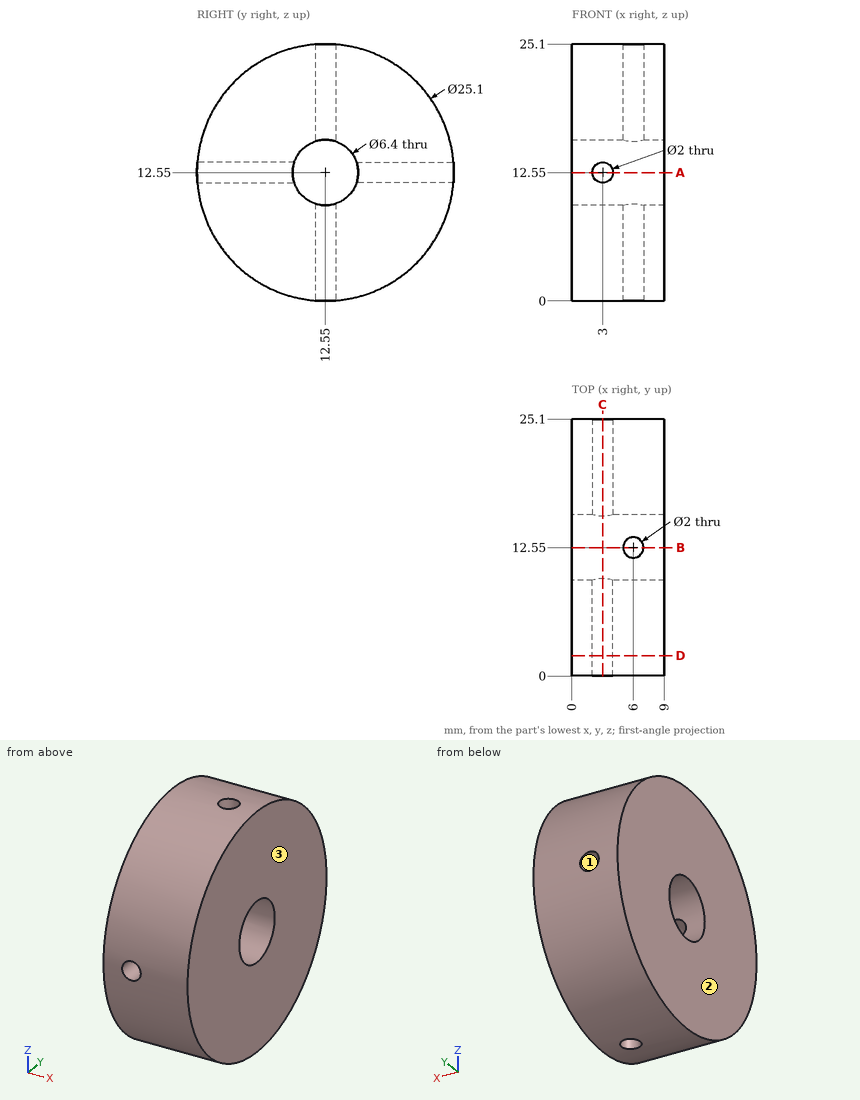
Input: dimensioned drawing with shaded views. Units: mm. Origin: part minimum x, y, z. Give positions to 0.01 mm unless a question says otherwise; leave off trailing zeros. Write each loop counter-clockwise with the first axis right and the second up, starting at its lowest first coordinate (ties: lowest second). Pieces come first, ordered by that corner, then holes.
Q1. First-contact query: P1, Ø2.5, axis at x = 6, y = 12.55, coming from the -Z side; P2, Ø4, axis at x = 7, z = 22, coming from the -Y side; P3, Ø1, axis at x = 1.5, y = 21, coming from the +Z side; P4, Ø1.5, axis at x = 1.5, z = 20, coming from the +Y side. Flat tips, straight axial feed; report the tip coordinate or a pass-through.
Q2. Material intervals for probe 1 along X at (y, z) = (5, 12.55); probe 2 along Y at (x, z) = (7.25, 12.55), sorted ascending.
Q3. Section A-A, the plane z = 12.55. Output: boundary loops of the cut face in (x, y).
Q4. Pull-direction query (X, two-part tool) for the marked faces 1, 2 and 3; classes: pulls with the +X half, pulls with the -X half, needs draft (parallel to the pull), parting line crosses it, or undercut.
Q5. Section C-C, the plane x = 3. Output: boundary loops of the cut face in (y, z).
Q6. Section B-B, the plane y = 12.55. Output: boundary loops of the cut face in (x, z).
Q7. Section D-D, the plane y = 2. Output: boundary loops of the cut face in (x, z), plus the area to 3 significant figures.
Filled in:
1. P1: stops at z = 0
1. P2: stops at y = 2.45
1. P3: stops at z = 22.26
1. P4: stops at y = 23.16
2. probe 1: x = 0 to 2, 4 to 9
2. probe 2: y = 0 to 9.35, 15.75 to 25.1
3. outline: (0, 0) - (2, 0) - (2, 9.35) - (0, 9.35) - close; (0, 15.75) - (2, 15.75) - (2, 25.1) - (0, 25.1) - close; (4, 0) - (9, 0) - (9, 9.35) - (4, 9.35) - close; (4, 15.75) - (9, 15.75) - (9, 25.1) - (4, 25.1) - close
4. face 1: undercut
4. face 2: pulls with the -X half
4. face 3: pulls with the +X half
5. outline: (0.04, 11.55) arc R12.55 ccw to (25.06, 11.55) - (15.59, 11.55) arc R3.2 cw to (9.51, 11.55) - close; (0.04, 13.55) - (9.51, 13.55) arc R3.2 cw to (15.59, 13.55) - (25.06, 13.55) arc R12.55 ccw to start
6. outline: (0, 0) - (5, 0) - (5, 9.35) - (0, 9.35) - close; (0, 15.75) - (5, 15.75) - (5, 25.1) - (0, 25.1) - close; (7, 0) - (9, 0) - (9, 9.35) - (7, 9.35) - close; (7, 15.75) - (9, 15.75) - (9, 25.1) - (7, 25.1) - close
7. outline: (0, 5.75) - (9, 5.75) - (9, 19.35) - (0, 19.35) - close; hole circle Ø2 at (3, 12.55)
7. area: 119 mm2
